Autodesk Inventor part; units mm, degrees
ref_plane "YZ Plane" through (0, 0, 0) normal (1, 0, 0) x (0, 1, 0)
ref_plane "XZ Plane" through (0, 0, 0) normal (0, 1, 0) x (-1, 0, 0)
ref_plane "XY Plane" through (0, 0, 0) normal (0, 0, 1) x (1, 0, 0)
sketch "Sketch2" plane through (0, 0, 0) normal (0, 1, 0) x (-1, 0, 0)
  circle A0 centre (0, 0) radius 37.5
  circle A1 centre (0, 0) radius 46.5
  line L0 (26.5165, -26.5165) -> (32.8805, -32.8805)
  line L1 (0, 0) -> (46.5, 0) construction
  circle A2 centre (29.6985, -29.6985) radius 1.5
  dimension "d14" = 75
  dimension "d15" = 9
  dimension "d25" = 45
  dimension "d26" = 9
  dimension "d27" = 3
extrude "Extrusion1" add sketch "Sketch2" along normal blind 1 contours A1 | A2 L0 | L0 A2
sketch "Sketch3" plane through (0, 1, 0) normal (0, 1, 0) x (1, 0, 0)
  circle A0 centre (0, 0) radius 46.5
  line L0 (-46.5, 0) -> (-37.5, 0)
  circle A1 centre (0, 0) radius 37.5
  circle A2 centre (0, 0) radius 42
  point P0 (-42, 0)
  point P1 (42, 0)
  point P2 (0, 42)
  point P3 (0, -42)
hole "Hole1" at (-42, 1, 0) at (42, 1, 0) at (0, 1, -42) at (0, 1, 42) direction (0, -1, 0) diameter 3.242 depth 11.8
extrude "Extrusion2" cut sketch "Sketch2" along normal blind 0.25 contours A2 L0 | L0 A2
pattern_circular "Circular Pattern1" count 20 over 360 about axis through (0, -10, 0) along (0, 1, 0) of "Extrusion2"
properties part number "LightPoint_LedStripMetal"
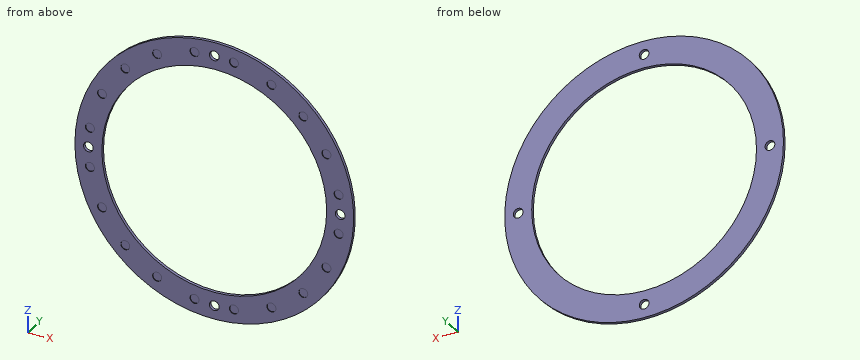
Source: CAD feature listing. Evaluate the final solid. Frame: model axes, mm. Coordinates: 2 decimals unless noted, no trailing zeros. Loops run counter-clockwise (first coordinate to the right, second up) from the corner with the lowest first, then second, coordinate; pieces in that order, holes last. Notation, with made-up numbers: M 10,19.25 L 56,19.25 A20 ccw 56,29.25 Z; hole C 56,87.5 d1. An arc over 180 degrees is marked long. Put each result on its own line as item: value. Start each with the question number.
1) Cut plane A-A on x = 0. Return the cut outline in (y, z).
2) Contact query for flat-ended pins moving along their axis: pin 1 Ø0.9 at (x, z) = (-7, -42) entering from -Y; pin 2 Ø1.9 at (x, z) = (0, -42) entering from +Y. Output: stop coordinate, or through.
3) Cut plane D-D on z = 10. Return the cut outline in (x, y), then the cut area to 3 significant figures.
4) Cut plane B-B on z = 0. Return the cut outline in (x, y), then the cut area to 3 significant figures.
5) Ray query, L1, parallel to Z at x = 0, y = 0.75; L2, parallel to Z at x = -1, y = 0.95; L3, parallel to X at y = 0.65, z = -30. Return the intervals inside material, ascending. Write a range as from..to.
6) Cut plane C-C on y = 0.6. Return the cut outline in (x, z), then the cut area to 3 significant figures.
The answers:
1. outline: M 0,-46.5 L 1,-46.5 L 1,-43.62 L 0,-43.62 Z; M 0,-40.38 L 1,-40.38 L 1,-37.5 L 0,-37.5 Z; M 0,37.5 L 1,37.5 L 1,40.38 L 0,40.38 Z; M 0,43.62 L 1,43.62 L 1,46.5 L 0,46.5 Z
2. pin 1: stops at y = 0.25
2. pin 2: passes through
3. outline: M -45.41,0 L -36.14,0 L -36.14,1 L -45.41,1 Z; M 36.14,0 L 45.41,0 L 45.41,1 L 36.14,1 Z
3. area: 18.5 mm²
4. outline: M -46.5,0 L -43.62,0 L -43.62,1 L -46.5,1 Z; M -40.38,0 L -37.5,0 L -37.5,1 L -40.38,1 Z; M 37.5,0 L 40.38,0 L 40.38,1 L 37.5,1 Z; M 43.62,0 L 46.5,0 L 46.5,1 L 43.62,1 Z
4. area: 11.5 mm²
5. L1: z = -46.5..-43.62, -40.38..-37.5, 37.5..40.38, 43.62..46.5
5. L2: z = -46.49..-43.28, -40.72..-37.49, 37.49..40.72, 43.28..46.49
5. L3: x = -35.53..-22.5, 22.5..35.53
6. outline: C 0,0 d93; hole C -42,0 d3.24; hole C 0,0 d75; hole C 0,-42 d3.24; hole C 0,42 d3.24; hole C 42,0 d3.24
6. area: 2,340 mm²
